Can you work these out from the model? Positions are in its coordinate system, mm. Give positions to 0.01 mm unless a question says otherwise; leave off trailing zeros. Order: outer loops, then holes, each group sorted by start corner. A loop starts at its lowest first (then second) coordinate and runs counter-clockwise, first axis right, second up. Notation, with made-up numbers: (-37, -22) -> (9, -22) arc R21 ccw to (9, -15) -> close; hole circle Ø8 at (41, 43). An arc over 180 degrees is marked (long way). Answer as a JSON object with one key per item and string values.
```python
from build123d import *

# Parameters (mm, degrees)
SKETCH1_W           = 88.9
SKETCH1_H           = 304.8
SKETCH1_W_2         = 63.5
SKETCH1_H_2         = 279.4
BOSS_EXTRUDE1_DEPTH = 3.175
SKETCH7_R           = 2.159
CUT_EXTRUDE2_DEPTH  = 159.781746826
FILLET1_R           = 12.7
FILLET3_R           = 3.175


with BuildPart() as part:
    # Sketch1 → Boss-Extrude1 (new body)
    with BuildSketch(Plane(origin=(0, 0, 0), x_dir=(1, 0, 0), z_dir=(0, 1, 0))):
        Rectangle(SKETCH1_W, SKETCH1_H)
        Rectangle(SKETCH1_W_2, SKETCH1_H_2, mode=Mode.SUBTRACT)
    extrude(amount=BOSS_EXTRUDE1_DEPTH)

    # Sketch7 → Cut-Extrude2 (cut, through all)
    with BuildSketch(Plane(origin=(0, 3.175, 0), x_dir=(1, 0, 0), z_dir=(0, 1, 0))):
        with Locations(Location((-38.1, 146.05, 0), (0, 0, 270))):
            Circle(SKETCH7_R)
        with Locations(Location((-38.1, 73.025, 0), (0, 0, 270))):
            Circle(SKETCH7_R)
        with Locations(Location((-38.1, 0, 0), (0, 0, 270))):
            Circle(SKETCH7_R)
        with Locations(Location((-38.1, -73.025, 0), (0, 0, 270))):
            Circle(SKETCH7_R)
        with Locations(Location((-38.1, -146.05, 0), (0, 0, 270))):
            Circle(SKETCH7_R)
        with Locations(Location((38.1, -146.05, 0), (0, 0, 90))):
            Circle(SKETCH7_R)
        with Locations(Location((38.1, -73.025, 0), (0, 0, 90))):
            Circle(SKETCH7_R)
        with Locations(Location((38.1, 0, 0), (0, 0, 90))):
            Circle(SKETCH7_R)
        with Locations(Location((38.1, 73.025, 0), (0, 0, 90))):
            Circle(SKETCH7_R)
        with Locations(Location((38.1, 146.05, 0), (0, 0, 90))):
            Circle(SKETCH7_R)
        with Locations(Location((0, 146.05, 0), (0, 0, 270))):
            Circle(SKETCH7_R)
        with Locations(Location((0, -146.05, 0), (0, 0, 90))):
            Circle(SKETCH7_R)
    extrude(amount=-CUT_EXTRUDE2_DEPTH, mode=Mode.SUBTRACT)

    # Fillet1
    fillet1_edges = [part.edges().sort_by_distance(p)[0] for p in [
        (-31.75, 1.5875, -139.7),
        (-31.75, 1.5875, 139.7),
        (31.75, 1.5875, 139.7),
        (31.75, 1.5875, -139.7),
    ]]
    fillet(fillet1_edges, radius=FILLET1_R)

    # Fillet3
    fillet3_edges = [part.edges().sort_by_distance(p)[0] for p in [
        (-44.45, 1.5875, -152.4),
        (44.45, 1.5875, -152.4),
        (44.45, 1.5875, 152.4),
        (-44.45, 1.5875, 152.4),
    ]]
    fillet(fillet3_edges, radius=FILLET3_R)


solid = part.part
```
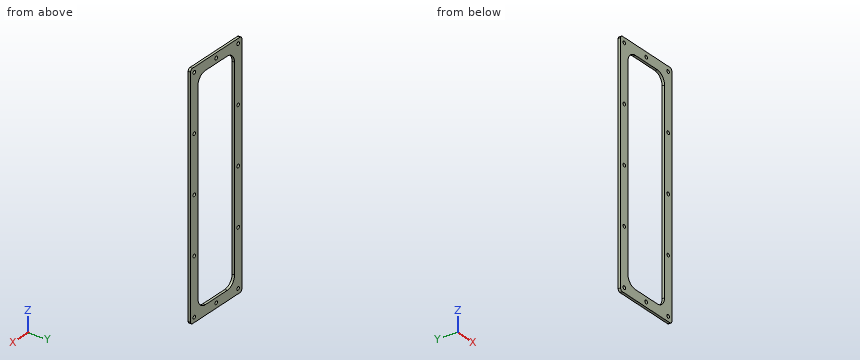
1. Will these pins go through, and if not, where does the flat tip stop? pin 1 Ø7 at (x, z) = (38.1, -146.05) entering from +Y (3 decimals); pin 2 Ø3.5 at (x, z) = (38.1, -73.025) entering from +Y.
Worked answers:
{"pin 1": "y = 3.175", "pin 2": "through"}
2. If we section it at A-A on x = 16: Please give me the cut outline in (y, z) (3 decimals), then the cut area to 3 significant figures.
Worked answers:
{"outline": "(0, -152.4) -> (3.175, -152.4) -> (3.175, -139.7) -> (0, -139.7) -> close; (0, 139.7) -> (3.175, 139.7) -> (3.175, 152.4) -> (0, 152.4) -> close", "area": "80.6 mm²"}
3. If we section it at B-B on z = 24: Please give me the cut outline in (x, y) (3 decimals).
Worked answers:
{"outline": "(-44.45, 0) -> (-31.75, 0) -> (-31.75, 3.175) -> (-44.45, 3.175) -> close; (31.75, 0) -> (44.45, 0) -> (44.45, 3.175) -> (31.75, 3.175) -> close"}
4. If we section it at C-C on y = 0.5: Count the separate pieces of the cut face and the enclosed holes in it, then the cut area to 3 significant figures.
Worked answers:
{"separate pieces": "1", "enclosed holes": "13", "area": "9,310 mm²"}
5. Please list where these lines run through material, in increasing order: L1, parallel to Z at x = -38, y = 2.45; L2, parallel to X at y = 1.5, z = 146.05; L3, parallel to X at y = 1.95, z = 0.
Worked answers:
{"L1": "-152.4 to -148.21, -143.89 to -75.18, -70.87 to -2.16, 2.16 to 70.87, 75.18 to 143.89, 148.21 to 152.4", "L2": "-44.45 to -40.26, -35.94 to -2.16, 2.16 to 35.94, 40.26 to 44.45", "L3": "-44.45 to -40.26, -35.94 to -31.75, 31.75 to 35.94, 40.26 to 44.45"}
